```python
from build123d import *

# Parameters (mm, degrees)
F0_R     = 7.0954565199
F1_DEPTH = 4.826
F2_DEPTH = 4.5466


# Not quite as in the source:
# - the program builds the solid bodies; features that only make, move or delete a surface that nothing else refers to are left out


with BuildPart() as f1:
    # F0 (on Top) → F1 (new body, symmetric)
    with BuildSketch(Plane.XY):
        Circle(F0_R)
        with BuildLine():
            ThreePointArc((3.3010527039, 3.9012801832), (4.4504568739, 2.5120449112), (5.045856518, 0.8101037104))
            ThreePointArc((5.045856518, 0.8101037104), (5.0942933944, 0.4063383238), (5.1104731701, 0))
            ThreePointArc((5.1104731701, 0), (4.6361016651, -2.1502319347), (3.3010527039, -3.9012801832))
            ThreePointArc((3.3010527039, -3.9012801832), (0, -5.1104731701), (-3.3010527039, -3.9012801832))
            ThreePointArc((-3.3010527039, -3.9012801832), (-4.7923906287, -1.7748036747), (-5.045856518, 0.8101037104))
            ThreePointArc((-5.045856518, 0.8101037104), (-4.4504568739, 2.5120449112), (-3.3010527039, 3.9012801832))
            ThreePointArc((-3.3010527039, 3.9012801832), (0, 5.1104731701), (3.3010527039, 3.9012801832))
        make_face(mode=Mode.SUBTRACT)
    extrude(amount=F1_DEPTH, both=True)

    # F0 (on Top) → F2 (join, symmetric)
    with BuildSketch(Plane.XY):
        with BuildLine():
            ThreePointArc((0.3718910489, 0.4422755592), (0.5238357878, 0.243939931), (0.57785, 0))
            Line((0.57785, 0), (5.045856518, 0.8101037104))
            ThreePointArc((5.045856518, 0.8101037104), (4.4504568739, 2.5120449112), (3.3010527039, 3.9012801832))
            Line((3.3010527039, 3.9012801832), (0.3718910489, 0.4422755592))
        make_face()
        with BuildLine():
            ThreePointArc((-0.57785, 0), (-0.5238357878, 0.243939931), (-0.3718910489, 0.4422755592))
            Line((-0.3718910489, 0.4422755592), (-3.3010527039, 3.9012801832))
            ThreePointArc((-3.3010527039, 3.9012801832), (-4.4504568739, 2.5120449112), (-5.045856518, 0.8101037104))
            Line((-5.045856518, 0.8101037104), (-0.57785, 0))
        make_face()
        with BuildLine():
            Line((3.3010527039, -3.9012801832), (0.3718910489, -0.4422755592))
            ThreePointArc((0.3718910489, -0.4422755592), (0, -0.57785), (-0.3718910489, -0.4422755592))
            Line((-0.3718910489, -0.4422755592), (-3.3010527039, -3.9012801832))
            ThreePointArc((-3.3010527039, -3.9012801832), (0, -5.1104731701), (3.3010527039, -3.9012801832))
        make_face()
    extrude(amount=F2_DEPTH, both=True)


solid = f1.part
```
Could you check a few things on this model? Use its own coordinates, in mm. A direction names the side the tool comes from. Round coordinates to 2 decimals unless told otherwise and drop trailing zeros. Loops run counter-clockwise (first coordinate to the right, second up) from the corner with the lowest first, then second, coordinate; pieces in that order, holes last.
Q1. I want a section at A-A (x = 0). Write out the boundary of the cut face in (y, z), and give its area (3 significant figures).
Q2. Please list where these lines run through material, in increasing order: L1, parallel to X at y = -3.5, z = 4; L2, parallel to X at y = -3.75, z = -1.75; L3, parallel to Y at x = -1.75, z = -1.75.
Q3. For P1, Ø2, axis at y = -3, z = 0, coming from the -X side; P2, Ø4.5, axis at x = 3, y = 1, coming from the +Z side; P3, Ø2, axis at x = -2, y = 1, coming from the -Z side; P4, Ø1.5, axis at y = -2, z = 1, coming from the +X side, each with a flat end and sliding along its axis, tell me the tip position at first contact or that it passes through.
Q4. I want a section at C-C (y = 4.5). Write out the boundary of the cut face in (x, z), and give its area (3 significant figures).
Q5. Thinking about a two-plate mould opening in X: for faces 5 (the cylindrical face through (-1.538, -6.927, 0.068)), 6 (the flat face through (-3, 2, 4.547)), 7 (the flat face through (-5, 2, 4.826)), which applies, pulls with the +X half, pulls with the -X half, needs draft (parallel to the pull), parting line crosses it, or undercut?
Q6. I want a section at B-B (z = 4.25). Write out the boundary of the cut face in (x, y).
Q7. On a 3-axis mill with a long thin cutter (end or side, diameter ignored), from which of +Z, -Z, +X, -X, +Y, -Y can I reach the whole of each face in a straight line? I mean faces 1 (the flat face through (0, -3, 4.547)), 2 (the flat face through (3, 2, -4.547)), 3 (the flat face through (-1.82, -2.15, 0.06)), 4 (the flat face through (-5, 2, -4.826)). Say none if no direction works.
Q8. I want a section at D-D (y = -1.75). Write out the boundary of the cut face in (x, z), and give its area (3 significant figures).
Answer below:
1. outline: (-7.1, -4.83) - (-5.11, -4.83) - (-5.11, -4.55) - (-0.58, -4.55) - (-0.58, 4.55) - (-5.11, 4.55) - (-5.11, 4.83) - (-7.1, 4.83) - close; (5.11, -4.83) - (7.1, -4.83) - (7.1, 4.83) - (5.11, 4.83) - close
1. area: 79.5 mm2
2. L1: x = -6.17 to -3.72, -2.96 to 2.96, 3.72 to 6.17
2. L2: x = -6.02 to -3.47, -3.17 to 3.17, 3.47 to 6.02
2. L3: y = -6.88 to -2.07, 0.21 to 2.07, 4.8 to 6.88
3. P1: stops at x = -6.81
3. P2: stops at z = 4.83
3. P3: stops at z = -4.55
3. P4: stops at x = 6.98
4. outline: (-5.49, -4.83) - (-2.42, -4.83) - (-2.42, 4.83) - (-5.49, 4.83) - close; (2.42, -4.83) - (5.49, -4.83) - (5.49, 4.83) - (2.42, 4.83) - close
4. area: 59.1 mm2
5. face 5: parting line crosses it
5. face 6: undercut
5. face 7: needs draft
6. outline: circle Ø14.19 at (0, 0); hole (-5.05, 0.81) arc R5.11 ccw to (-3.3, -3.9) - (-0.37, -0.44) arc R0.58 ccw to (0.37, -0.44) - (3.3, -3.9) arc R5.11 ccw to (5.05, 0.81) - (0.58, 0) arc R0.58 ccw to (0.37, 0.44) - (3.3, 3.9) arc R5.11 ccw to (-3.3, 3.9) - (-0.37, 0.44) arc R0.58 ccw to (-0.58, 0) - close
7. face 1: +Z
7. face 2: -Z
7. face 3: +Z, -Z
7. face 4: -Z, +X, -X, +Y, -Y
8. outline: (-6.88, -4.83) - (-4.8, -4.83) - (-4.8, 4.83) - (-6.88, 4.83) - close; (-1.48, -4.55) - (1.48, -4.55) - (1.48, 4.55) - (-1.48, 4.55) - close; (4.8, -4.83) - (6.88, -4.83) - (6.88, 4.83) - (4.8, 4.83) - close
8. area: 67.0 mm2
